```python
from build123d import *

# Parameters (mm, degrees)
SKETCH1_R           = 2
BOSS_EXTRUDE1_DEPTH = 8
CUT_EXTRUDE1_START  = 17.721034
SKETCH2_R           = 1
CUT_EXTRUDE1_DEPTH  = 8
FILLET1_R           = 2


with BuildPart() as part:
    # Sketch1 → Boss-Extrude1 (new body)
    with BuildSketch(Plane(origin=(0, 0, 0), x_dir=(1, 0, 0), z_dir=(0, 1, 0))):
        Polygon((19.047511312, 22.278966214), (33.547511312, 22.278966214), (33.547511312, -17.721033786), (-34.452488688, -17.721033786), (-34.452488688, 22.278966214), (-21.952488688, 22.278966214), (-21.952488688, 2.278966214), (19.047511312, 2.278966214), align=None)
        with Locations(Location((-25.452488688, 18.278966214, 0), (0, 0, 270))):
            Circle(SKETCH1_R, mode=Mode.SUBTRACT)
        with Locations(Location((-25.452488688, 6.278966214, 0), (0, 0, 270))):
            Circle(SKETCH1_R, mode=Mode.SUBTRACT)
        with Locations(Location((22.547511312, 18.278966214, 0), (0, 0, 270))):
            Circle(SKETCH1_R, mode=Mode.SUBTRACT)
        with Locations(Location((22.547511312, 6.278966214, 0), (0, 0, 270))):
            Circle(SKETCH1_R, mode=Mode.SUBTRACT)
    extrude(amount=BOSS_EXTRUDE1_DEPTH)

    # Sketch2 → Cut-Extrude1 (cut)
    with BuildSketch(Plane.XY.offset(CUT_EXTRUDE1_START)):
        with Locations(Location((-24.452488688, 4, 0), (0, 0, 180))):
            Circle(SKETCH2_R)
        with Locations(Location((23.547511312, 4, 0), (0, 0, 180))):
            Circle(SKETCH2_R)
    extrude(amount=-CUT_EXTRUDE1_DEPTH, mode=Mode.SUBTRACT)

    # Fillet1
    # the kernel refuses this fillet: 2 mm, written as the material it takes off along each edge
    with BuildSketch(Plane(origin=(19.047511312, 8, -2.278966214), x_dir=(0, -1, 0), z_dir=(0, 0, -1))) as fillet1_piece_1:
        with BuildLine():
            CenterArc((FILLET1_R, -FILLET1_R), FILLET1_R, 90, 90)
            Line((0, -FILLET1_R), (0, 0))
            Line((0, 0), (FILLET1_R, 0))
        make_face()
    extrude(amount=25, mode=Mode.SUBTRACT)
    with BuildSketch(Plane(origin=(-21.952488688, 8, -27.278966214), x_dir=(-1, 0, 0), z_dir=(0, 0, 1))) as fillet1_piece_2:
        with BuildLine():
            CenterArc((FILLET1_R, FILLET1_R), FILLET1_R, 180, 90)
            Line((0, FILLET1_R), (0, 0))
            Line((0, 0), (FILLET1_R, 0))
        make_face()
    extrude(amount=25, mode=Mode.SUBTRACT)


solid = part.part
```
Here's how the part is built. I have some questions about the finished solid (model axes, mm). A direction names the side the tool comes from. Round coordinates to 2 decimals unless told otherwise and drop trailing zeros. Write each loop counter-clockwise with the first axis right and the second up, starting at its lowest first coordinate (ties: lowest second). Pieces come first, ordered by that corner, then holes.
Q1. If we section it at B-B on x = -19.5: Write out the boundary of the cut face in (y, z).
Q2. If we section it at A-A on y = 4: Write out the boundary of the cut face in (x, z).
Q3. If we mould it in two halves opening along Y, with no side actions, what happens to faces 1 (the cylindrical face through (22.594, 3.7, 13.777)), 2 (the flat face through (-34.452, 4, -2)), 3 (the cylindrical face through (19.62, 7.4, -12.14))? For each: +Y half, -Y half, draft (parallel to the pull), parting line (faces both ways), or undercut.
Q4. Will these pins go through, and if not, where does the flat tip stop? P1, Ø2.5, axis at x = 22.55, z = -6.28, coming from the -Y side; P2, Ø3, axis at x = 13.5, y = 7, coming from the -Z side.
Q5. Please list where these lines run through material, in increasing order: probe 1 along X at (y, z) = (4, 11.5); probe 2 along X at (y, z) = (1, -13); probe 3 along Z at (x, y) = (-24, 2.25).
Q6. Which directions (+Z, -Z, +X, -X, +Y, -Y) give clear straight access to the entire face, cutting with the end or side of a thin tool? Please do faces 4 (the flat face through (-24, 4, 9.721)), 5 (the flat face through (26, 4, -22.279)), 6 (the flat face through (-21.952, 3, -12)), 7 (the cylindrical face through (-22.523, 7.399, -12.419)).
Answer below:
1. outline: (0, -2.28) - (8, -2.28) - (8, 17.72) - (0, 17.72) - close
2. outline: (-34.45, -22.28) - (-21.95, -22.28) - (-21.95, -2.28) - (19.05, -2.28) - (19.05, -22.28) - (33.55, -22.28) - (33.55, 17.72) - (24.55, 17.72) - (24.55, 9.72) - (22.55, 9.72) - (22.55, 17.72) - (-23.45, 17.72) - (-23.45, 9.72) - (-25.45, 9.72) - (-25.45, 17.72) - (-34.45, 17.72) - close; hole circle Ø4 at (-25.45, -18.28); hole circle Ø4 at (-25.45, -6.28); hole circle Ø4 at (22.55, -18.28); hole circle Ø4 at (22.55, -6.28)
3. face 1: undercut
3. face 2: draft
3. face 3: +Y half
4. P1: passes through
4. P2: stops at z = -2.28
5. probe 1: x = -34.45 to -25.45, -23.45 to 22.55, 24.55 to 33.55
5. probe 2: x = -34.45 to -21.95, 19.05 to 33.55
5. probe 3: z = -22.28 to -19.65, -16.9 to -7.65, -4.9 to 17.72
6. face 4: +Z
6. face 5: -Z, +X, -X, +Y, -Y
6. face 6: -Z, +Y, -Y
6. face 7: -Z, +Y
